```python
from build123d import *

# Parameters (mm, degrees)
BOSS_EXTRUDE1_DEPTH = 1600


with BuildPart() as part:
    # Sketch1 → Boss-Extrude1 (new body)
    with BuildSketch(Plane.XY):
        with BuildLine():
            Line((1897.37, 0), (1987.30887071, -116.111138292))
            Line((1987.30887071, -116.111138292), (1979.403162377, -122.234844339))
            Line((1979.403162377, -122.234844339), (1889.464291667, -6.123706047))
            ThreePointArc((1889.464291667, -6.123706047), (948.685, 455.155274378), (7.905708333, -6.123706047))
            Line((7.905708333, -6.123706047), (6.326316618, -8.167278707))
            Line((6.326316618, -8.167278707), (0, 0))
            ThreePointArc((0, 0), (948.685, 465.155274378), (1897.37, 0))
        make_face()
    extrude(amount=BOSS_EXTRUDE1_DEPTH)


solid = part.part
```
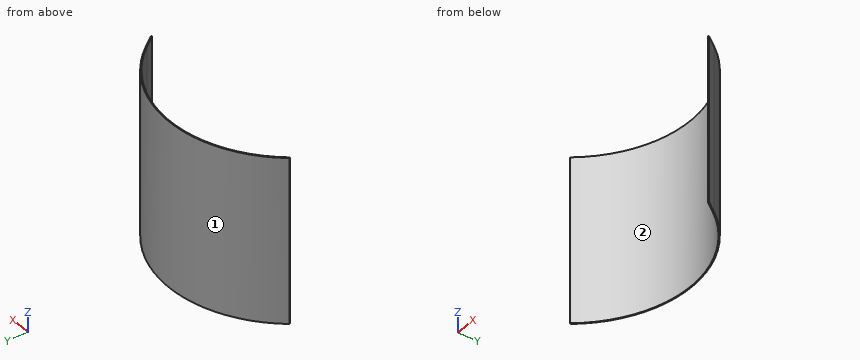
Verification items for the finished model (mm, model axes). Face numbers are marked on the shaded views. Round coordinates to 2 decimals unless told otherwise and drop trailing zeros. Order: outer loops, then holes, each group sorted by start corner. A loop starts at its lowest first (then second) coordinate and runs counter-clockwise, first axis right, second up.
1) Draft check along X on the marked faces 1 and 2. Enter one of: +X half, -X half, draft (parallel to the pull), parting line (faces both ways), or undercut.
Geometry says:
face 1: parting line
face 2: undercut
2) Material ranges on line 1 (X direction, y = 323, z = 531); line 2 (X direction, y = 365, z = 1220); line 3 (Y direction, x = 966.5, z = 1191), recorded low to high.
Geometry says:
line 1: x = 382.15 to 403.65, 1493.72 to 1515.22
line 2: x = 468.75 to 494.33, 1403.04 to 1428.62
line 3: y = 455.02 to 465.02
3) Cross-section at B-B, the plane z = 1365. Record the cut outline in (x, y) (3 decimals).
Geometry says:
outline: (0, 0) - (6.326, -8.167) - (7.906, -6.124) arc R1190 cw to (1889.464, -6.124) - (1979.403, -122.235) - (1987.309, -116.111) - (1897.37, 0) arc R1200 ccw to start
4) Cross-section at D-D, the plane x = 1616. Record the cut outline in (y, z).
Geometry says:
outline: (250.44, 0) - (262.5, 0) - (262.5, 1600) - (250.44, 1600) - close
5) Depth check by flat-ended pin: pin 1 (12 mm diameter, centred on x = 428, z = 1313, fed in from -Y); pin 2 (12 mm diameter, centred on x = 346, z = 532, fed in from +Y); pin 3 (12 mm diameter, centred on y = 95, z = 834.5, fed in from -X); pin 4 (10 mm diameter, centred on x = 1753.5, y = 130.5, fed in from +Z). Enter the tip coordinate at first touch or a pass-through.
Geometry says:
pin 1: stops at y = 332.26
pin 2: stops at y = 306.29
pin 3: stops at x = 76.17
pin 4: passes through
